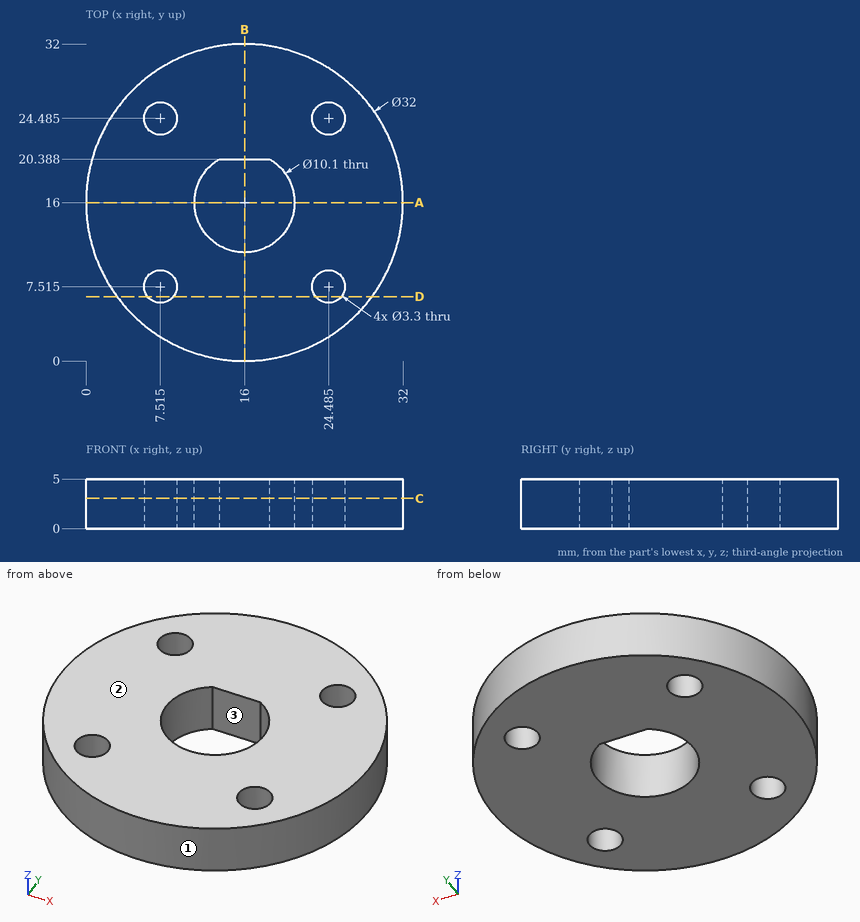
Verification items for this drawing (mm, ordinates from the low corner). Give positions to 0.01 mm unless a question says otherwise; leave off trailing zeros. Write each loop counter-clockwise with the first axis right and the second up, starting at its lowest first coordinate (ties: lowest second). Pieces come first, ordered by that corner, then holes. Notation, with made-up numbers: (44.25, -6.5) -> (98.25, -6.5) arc R23 ccw to (98.25, 9.5) -> close; hole circle Ø8 at (-28, -26.5). An arc over 180 degrees is marked (long way). Use CSV: the item, a comma, the result in double quotes.
(1) Sectioned sample at D-D (y = 6.5). Record the cut outline in (x, z), plus the area to 3 significant figures.
Derived:
outline,"(3.13, 0) -> (6.21, 0) -> (6.21, 5) -> (3.13, 5) -> close; (8.82, 0) -> (23.18, 0) -> (23.18, 5) -> (8.82, 5) -> close; (25.79, 0) -> (28.87, 0) -> (28.87, 5) -> (25.79, 5) -> close"
area,"103 mm^2"
(2) Sectioned sample at B-B (x = 16). Record the cut outline in (y, z).
Derived:
outline,"(0, 0) -> (10.95, 0) -> (10.95, 5) -> (0, 5) -> close; (20.39, 0) -> (32, 0) -> (32, 5) -> (20.39, 5) -> close"
(3) Release check for a two-part mould opening along X. For the marked faces 1, 2 and 3 record: +X half, -X half, draft (parallel to the pull), parting line (faces both ways), or undercut.
Derived:
face 1,"parting line"
face 2,"draft"
face 3,"undercut"
(4) Sectioned sample at C-C (z = 3.05). Give the number of separate pieces and of enclosed holes in the cut face, plus the area to 3 significant figures.
Derived:
separate pieces,"1"
enclosed holes,"5"
area,"692 mm^2"
(5) Go/stop test with flat-tipped pins: pin 1 (1.5 mm diameter, centred on y = 11.5, z = 1.5, fed in from +X); pin 2 (1.5 mm diameter, centred on x = 27.5, z = 4, fed in from +Y); pin 3 (3 mm diameter, centred on x = 7.51, y = 24.49, fed in from +Z). Record where each tip stops, or that it passes through.
Derived:
pin 1,"stops at x = 31.55"
pin 2,"stops at y = 27.85"
pin 3,"passes through"
(6) Material ranges on L1, parallel to Y at x = 16, z = 2; L2, parallel to Y at x = 26, z = 1.05; L3, parallel to Y at x = 24.5, z = 4.7 (1 decimal), recorded low to high.
Derived:
L1,"y = 0 to 10.95, 20.39 to 32"
L2,"y = 3.51 to 6.86, 8.17 to 23.83, 25.14 to 28.49"
L3,"y = 2.4 to 5.9, 9.2 to 22.8, 26.1 to 29.6"
(7) Sectioned sample at A-A (y = 16). Record the cut outline in (x, z), plus the area to 4 significant figures.
Derived:
outline,"(0, 0) -> (10.95, 0) -> (10.95, 5) -> (0, 5) -> close; (21.05, 0) -> (32, 0) -> (32, 5) -> (21.05, 5) -> close"
area,"109.5 mm^2"
